```python
from build123d import *

# Parameters (mm, degrees)
BOSS_EXTRUDE1_DEPTH     = 1.6
FILLET1_R               = 3
M2_CLEARANCE_HOLE1_D    = 2.6
CUT_EXTRUDE1_DEPTH      = 38.159251876
CUT_EXTRUDE1_DEPTH_BACK = 38.159251876
SKETCH5_R               = 0.8
SKETCH6_R               = 3
CUT_EXTRUDE2_DEPTH      = 0.001


with BuildPart() as part:
    # Sketch1 → Boss-Extrude1 (new body)
    with BuildSketch(Plane(origin=(0, 0, 0), x_dir=(1, 0, 0), z_dir=(0, 1, 0))):
        Polygon((-13.5, -10), (-13.5, 10), (13.5, 10), (13.5, -10), (26.5, -10), (26.5, -26), (-13.5, -26), align=None)
    extrude(amount=BOSS_EXTRUDE1_DEPTH)

    # Fillet1
    fillet1_edges = [part.edges().sort_by_distance(p)[0] for p in [
        (13.5, 0.8, 10),
    ]]
    fillet(fillet1_edges, radius=FILLET1_R)

    # M2 Clearance Hole1 (through all)
    with Locations(Plane(origin=(0, 1.6, 0), x_dir=(1, 0, 0), z_dir=(0, 1, 0))):
        with Locations((-0.4, -5.1)):
            Hole(M2_CLEARANCE_HOLE1_D / 2)

    # Sketch5 → Cut-Extrude1 (cut, two sides: drawn at the far end of the back side and taken through both)
    with BuildSketch(Plane(origin=(0, 1.6, 0), x_dir=(1, 0, 0), z_dir=(0, 1, 0)).offset(-CUT_EXTRUDE1_DEPTH_BACK)):
        with Locations(Location((-12.225, 2.9, 0), (0, 0, 270))):
            Circle(SKETCH5_R)
        with Locations(Location((3.625, 2.9, 0), (0, 0, 270))):
            Circle(SKETCH5_R)
    extrude(amount=CUT_EXTRUDE1_DEPTH + CUT_EXTRUDE1_DEPTH_BACK, mode=Mode.SUBTRACT)

    # Sketch6 → Cut-Extrude2 (cut)
    with BuildSketch(Plane.XZ):
        with Locations(Location((-0.4, 5.1, 0), (0, 0, 270))):
            Circle(SKETCH6_R)
    extrude(amount=-CUT_EXTRUDE2_DEPTH, mode=Mode.SUBTRACT)


solid = part.part
```
The model under review builds one solid part; all positions refer to its coordinate system, in mm. A direction names the side the tool comes from. Give positions to 0.01 mm unless a question says otherwise; leave off trailing zeros. Write each loop counter-clockwise with the first axis right and the second up, starting at its lowest first coordinate (ties: lowest second). Pieces come first, ordered by that corner, then holes. Notation, with made-up numbers: (40, 24) - (86, 24) arc R30 ccw to (86, 58) - close; hole circle Ø7 at (-1.5, -33.75). An arc over 180 degrees is marked (long way). Answer in a Markdown table with one row per item. Add a question column.
1. We need section D-D on y = 0.25. Write out the cut boundary in (x, z) (3 decimals).
2. Wall thickness on line 1 along X through (y, z) = (0.4, -2.9) (3 decimals); line 2 along Z through (x, y) = (-0.4, 0.35); line 3 along Z through (x, y) = (0, 1.05): over which ranges is each line inside the solid? List them lowest first. Write a range as [from, to].
3. We need section B-B on z = -2.9. Write out the cut boundary in (x, y) (3 decimals).
4. Draft analysis for pull direction X (two halves, no side actions). For faces 3 (the cylindrical face through (-11.43, 0.79, -3)), 4 (the flat face through (-13.5, 1, 8)), 5 (the flat face through (26.5, 1, 18)), 6 (the flat face through (7, 1, 26)), state which applies: +X half, -X half, draft (parallel to the pull), parting line (faces both ways), or undercut.
5. Tool access review of faces 1 (the cylindrical face through (2.844, 0.789, -3.073)), 2 (the flat face through (21, 1, 10)): name each direction out of +Z, -Z, +X, -X, +Y, -Y from which nothing blocks a thin tool from reaching the whole face with its end or side.
Ans:
| question | item | result |
|---|---|---|
| 1 | outline | (-13.5, -10) - (13.5, -10) - (13.5, 7) arc R3 cw to (16.5, 10) - (26.5, 10) - (26.5, 26) - (-13.5, 26) - close; hole circle Ø1.6 at (-12.225, -2.9); hole circle Ø2.6 at (-0.4, 5.1); hole circle Ø1.6 at (3.625, -2.9) |
| 2 | line 1 | x = [-13.5, -13.025], [-11.425, 2.825], [4.425, 13.5] |
| 2 | line 2 | z = [-10, 3.8], [6.4, 26] |
| 2 | line 3 | z = [-10, 3.86], [6.34, 26] |
| 3 | outline | (-13.5, 0) - (-13.025, 0) - (-13.025, 1.6) - (-13.5, 1.6) - close; (-11.425, 0) - (2.825, 0) - (2.825, 1.6) - (-11.425, 1.6) - close; (4.425, 0) - (13.5, 0) - (13.5, 1.6) - (4.425, 1.6) - close |
| 4 | face 3 | undercut |
| 4 | face 4 | -X half |
| 4 | face 5 | +X half |
| 4 | face 6 | draft |
| 5 | face 1 | +Y, -Y |
| 5 | face 2 | -Z, +X, +Y, -Y |
